```python
from build123d import *

# Parameters (mm, degrees)
SKETCH1_W           = 57.15
SKETCH1_H           = 25.4
BOSS_EXTRUDE1_DEPTH = 57.15
SKETCH2_W           = 25.4
SKETCH2_H           = 19.05
CUT_EXTRUDE1_DEPTH  = 85.719566807
CUT_EXTRUDE3_DEPTH  = 142.865944679
BOSS_EXTRUDE2_DEPTH = 19.05
SKETCH8_W           = 25.4
SKETCH8_H           = 76.2
CUT_EXTRUDE4_DEPTH  = 12.7


with BuildPart() as part:
    # Sketch1 → Boss-Extrude1 (new body)
    with BuildSketch(Plane(origin=(0, 0, 0), x_dir=(0, 0, -1), z_dir=(1, 0, 0))):
        with Locations((-28.575, 12.7)):
            Rectangle(SKETCH1_W, SKETCH1_H)
    extrude(amount=-BOSS_EXTRUDE1_DEPTH)

    # Sketch2 → Cut-Extrude1 (cut, through all)
    with BuildSketch(Plane(origin=(0, 25.4, 0), x_dir=(1, 0, 0), z_dir=(0, 1, 0))):
        with Locations((-12.7, -9.525)):
            Rectangle(SKETCH2_W, SKETCH2_H)
    extrude(amount=-CUT_EXTRUDE1_DEPTH, mode=Mode.SUBTRACT)

    # Sketch4 → Cut-Extrude3 (cut, through all, along a direction that is not the sketch's normal)
    with BuildSketch(Plane.XY.offset(57.15)):
        Polygon((-50.8, 25.4), (-25.4, 0), (0, 0), (0, 25.4), align=None)
    extrude(amount=-CUT_EXTRUDE3_DEPTH, dir=(-0.8, 0, 0.6), mode=Mode.SUBTRACT)

    # Sketch6 → Boss-Extrude2 (add)
    with BuildSketch(Plane.ZY.offset(57.15)):
        Polygon((0, 0), (0, 50.8), (12.7, 50.8), (12.7, 41.275), (44.45, 41.275), (44.45, 50.8), (57.15, 50.8), (57.15, 0), align=None)
    extrude(amount=BOSS_EXTRUDE2_DEPTH)

    # Sketch8 → Cut-Extrude4 (cut)
    with BuildSketch(Plane(origin=(0, 25.4, 0), x_dir=(1, 0, 0), z_dir=(0, 1, 0))):
        with Locations((-12.7, -57.15)):
            Rectangle(SKETCH8_W, SKETCH8_H)
    extrude(amount=-CUT_EXTRUDE4_DEPTH, mode=Mode.SUBTRACT)


solid = part.part
```
Design review of the part built by this model. Coordinates are the model's own, in mm. A direction names the side the tool comes from. Give positions to 0.01 mm unless a question says otherwise; leave off trailing zeros. Order: outer loops, then holes, each group sorted by start corner. A loop starts at its lowest first (then second) coordinate and runs counter-clockwise, first axis right, second up. Notation, with made-up numbers: (45.5, 61.5) - (58.5, 61.5) arc R28 ccw to (58.5, 95.5) - close; hole circle Ø9 at (52.5, 51). An arc over 180 degrees is marked (long way). Use a Markdown table: item, result. Add a question column.
(1) Mouldability with a two-part tool opening along Z and no side actions: class faces 1 (the face through (-20.5, 9.7, 46.2)), 2 (the face through (-67, 46, 44.45)), 3 (the face through (-67, 41.275, 28)), 4 (the face through (0, 6, 27)) as +Z half, -Z half, draft (parallel to the pull), parting line (faces both ways), or undercut.
(2) Clearance check with flat-ended pins moving along their axes: P1, Ø12.5, axis at y = 34.5, z = 29, coming from the +X side; P2, Ø15, axis at x = -70.5, z = 35, coming from the +Y side (3 decimals); P3, Ø5, axis at x = -30, z = 30, coming from the +Y side; P4, Ø3, axis at x = -64, y = 47.5, coming from the -Z side. State where each tip first meets the part, or that it passes through.
(3) Machinability: for faces 5 (the face through (-41, 25.4, 23)), 6 (the face through (-13, 6, 19.05)), 7 (the face through (-76.2, 26, 29)), 8 (the face through (-67, 46, 12.7)), which of the approach directions +Z, -Z, +X, -X, +Y, -Y give a long, thin tool a straight path to every point of the face, cutting with its end or side? Answer none if there is none.
(4) Add section D-D on y = 9. Give the boundary of the cut face in (x, z).
(5) Wall thickness on probe 1 along Y at (x, z) = (-72, 20) (3 decimals); probe 2 along X at (y, z) = (17.5, 42); probe 3 along Y at (x, z) = (-42.5, 28): over which ranges is each line inside the solid? List them lowest first. Write a range as [from, to].
(6) Add section A-A on y = 46. Give the boundary of the cut face in (x, z), then the cut area to 3 significant figures.
(7) Add section B-B on z = 21.5. Give the boundary of the cut face in (x, y) (3 decimals).
(8) Add section C-C on x = -71. Give the boundary of the cut face in (y, z) (3 decimals).
Report:
| question | item | result |
|---|---|---|
| 1 | face 1 | +Z half |
| 1 | face 2 | undercut |
| 1 | face 3 | undercut |
| 1 | face 4 | draft |
| 2 | P1 | stops at x = -57.15 |
| 2 | P2 | stops at y = 41.275 |
| 2 | P3 | stops at y = 25.4 |
| 2 | P4 | stops at z = 0 |
| 3 | face 5 | +Z, -Z, +X, +Y |
| 3 | face 6 | -Z, +X, +Y, -Y |
| 3 | face 7 | +Z, -Z, -X, +Y, -Y |
| 3 | face 8 | +X, -X, +Y |
| 4 | outline | (-76.2, 0) - (-25.4, 0) - (-25.4, 19.05) - (0, 19.05) - (0, 31.35) - (-34.4, 57.15) - (-76.2, 57.15) - close |
| 5 | probe 1 | y = [0, 41.275] |
| 5 | probe 2 | x = [-76.2, -25.4] |
| 5 | probe 3 | y = [0, 25.4] |
| 6 | outline | (-76.2, 0) - (-57.15, 0) - (-57.15, 12.7) - (-76.2, 12.7) - close; (-76.2, 44.45) - (-57.15, 44.45) - (-57.15, 57.15) - (-76.2, 57.15) - close |
| 6 | area | 484 mm² |
| 7 | outline | (-76.2, 0) - (0, 0) - (0, 12.7) - (-25.4, 12.7) - (-25.4, 25.4) - (-57.15, 25.4) - (-57.15, 41.275) - (-76.2, 41.275) - close |
| 8 | outline | (0, 0) - (50.8, 0) - (50.8, 12.7) - (41.275, 12.7) - (41.275, 44.45) - (50.8, 44.45) - (50.8, 57.15) - (0, 57.15) - close |
